from build123d import *

# Parameters (mm, degrees)
SKETCH1_W            = 32.9
SKETCH1_H            = 32.9
SKETCH1_W_2          = 20.2
SKETCH1_H_2          = 20.2
BOSS_EXTRUDE1_DEPTH  = 25
M4_CLEARANCE_HOLE1_D = 4.5
M4_CLEARANCE_HOLE2_D = 4.5
SKETCH8_W            = 32.9
SKETCH8_H            = 32.9
SKETCH8_W_2          = 20.2
SKETCH8_H_2          = 20.2
BOSS_EXTRUDE2_DEPTH  = 12.7
SKETCH9_W            = 87.4
SKETCH9_H            = 82.4
BOSS_EXTRUDE3_DEPTH  = 6.35
M2_CLEARANCE_HOLE1_D = 2.4
SKETCH13_W           = 20.2
SKETCH13_H           = 20.2
CUT_EXTRUDE1_DEPTH   = 71.911353111
SKETCH14_W           = 87.4
SKETCH14_H           = 82.4
CUT_EXTRUDE2_DEPTH   = 75.481759512
SKETCH15_W           = 35
SKETCH15_H           = 35
SKETCH15_R           = 1.625
BOSS_EXTRUDE4_DEPTH  = 6.35
FILLET1_R            = 6.35
SKETCH16_W           = 8
SKETCH16_H           = 22
CUT_EXTRUDE3_DEPTH   = 95.077926699
FILLET2_R            = 3.175


with BuildPart() as part:
    # Sketch1 → Boss-Extrude1 (new body)
    with BuildSketch(Plane(origin=(0, 0, 0), x_dir=(1, 0, 0), z_dir=(0, 1, 0))):
        Rectangle(SKETCH1_W, SKETCH1_H)
        Rectangle(SKETCH1_W_2, SKETCH1_H_2, mode=Mode.SUBTRACT)
    extrude(amount=BOSS_EXTRUDE1_DEPTH)

    # M4 Clearance Hole1 (through all)
    with Locations(Plane.XY.offset(16.45)):
        with Locations((0, 12.5)):
            Hole(M4_CLEARANCE_HOLE1_D / 2)

    # M4 Clearance Hole2 (through all)
    with Locations(Plane(origin=(16.45, 0, 0), x_dir=(0, 0, -1), z_dir=(1, 0, 0))):
        with Locations((0, 12.5)):
            Hole(M4_CLEARANCE_HOLE2_D / 2)

    # Sketch8 → Boss-Extrude2 (add)
    with BuildSketch(Plane(origin=(0, 25, 0), x_dir=(1, 0, 0), z_dir=(0, 1, 0))):
        Rectangle(SKETCH8_W, SKETCH8_H)
        Rectangle(SKETCH8_W_2, SKETCH8_H_2, mode=Mode.SUBTRACT)
    extrude(amount=BOSS_EXTRUDE2_DEPTH)

    # Sketch9 → Boss-Extrude3 (add)
    with BuildSketch(Plane(origin=(0, 37.7, 0), x_dir=(1, 0, 0), z_dir=(0, 1, 0))):
        Rectangle(SKETCH9_W, SKETCH9_H)
    extrude(amount=BOSS_EXTRUDE3_DEPTH)

    # M2 Clearance Hole1 (through all)
    with Locations(Plane(origin=(0, 44.05, 0), x_dir=(1, 0, 0), z_dir=(0, 1, 0))):
        with Locations((35, -25), (-22, -31), (-22, 31), (35, 25)):
            Hole(M2_CLEARANCE_HOLE1_D / 2)

    # Sketch13 → Cut-Extrude1 (cut, through all)
    with BuildSketch(Plane.XZ.offset(-37.7)):
        Rectangle(SKETCH13_W, SKETCH13_H)
    extrude(amount=-CUT_EXTRUDE1_DEPTH, mode=Mode.SUBTRACT)

    # Sketch14 → Cut-Extrude2 (cut, through all)
    with BuildSketch(Plane(origin=(0, 44.05, 0), x_dir=(1, 0, 0), z_dir=(0, 1, 0))):
        Rectangle(SKETCH14_W, SKETCH14_H)
        with BuildLine():
            Line((40, 23.784646643), (40, -23.784646643))
            ThreePointArc((40, -23.784646643), (38.369303562, -28.033255108), (34.314748382, -30.099756269))
            Line((34.314748382, -30.099756269), (-19.985251618, -35.815545743))
            ThreePointArc((-19.985251618, -35.815545743), (-24.898608465, -34.219739679), (-27, -29.500436117))
            Line((-27, -29.500436117), (-27, 29.500436117))
            ThreePointArc((-27, 29.500436117), (-24.898608465, 34.219739679), (-19.985251618, 35.815545743))
            Line((-19.985251618, 35.815545743), (34.314748382, 30.099756269))
            ThreePointArc((34.314748382, 30.099756269), (38.369303562, 28.033255108), (40, 23.784646643))
        make_face(mode=Mode.SUBTRACT)
    extrude(amount=-CUT_EXTRUDE2_DEPTH, mode=Mode.SUBTRACT)

    # Sketch15 → Boss-Extrude4 (add)
    with BuildSketch(Plane(origin=(0, 44.05, 0), x_dir=(1, 0, 0), z_dir=(0, 1, 0))):
        with Locations((57.5, 0)):
            Rectangle(SKETCH15_W, SKETCH15_H)
        with Locations(Location((65, 7.5, 0), (0, 0, 270))):
            Circle(SKETCH15_R, mode=Mode.SUBTRACT)
        with Locations(Location((65, -7.5, 0), (0, 0, 270))):
            Circle(SKETCH15_R, mode=Mode.SUBTRACT)
    extrude(amount=-BOSS_EXTRUDE4_DEPTH)

    # Fillet1
    fillet1_edges = [part.edges().sort_by_distance(p)[0] for p in [
        (40, 40.875, 17.5),
        (40, 40.875, -17.5),
    ]]
    fillet(fillet1_edges, radius=FILLET1_R)

    # Sketch16 → Cut-Extrude3 (cut, through all)
    with BuildSketch(Plane(origin=(0, 44.05, 0), x_dir=(1, 0, 0), z_dir=(0, 1, 0))):
        with Locations((49, 0)):
            Rectangle(SKETCH16_W, SKETCH16_H)
    extrude(amount=-CUT_EXTRUDE3_DEPTH, mode=Mode.SUBTRACT)

    # Fillet2
    fillet2_edges = [part.edges().sort_by_distance(p)[0] for p in [
        (45, 40.875, 11),
        (45, 40.875, -11),
        (53, 40.875, -11),
        (53, 40.875, 11),
    ]]
    fillet(fillet2_edges, radius=FILLET2_R)


solid = part.part
Model file for the job. Use its own axes, mm. A direction names the side the tool comes from. Give positions to 0.01 mm unless a question says otherwise; leave off trailing zeros. Loops run counter-clockwise (first coordinate to the right, second up) from the corner with the lowest first, then second, coordinate; pieces in that order, holes last. Notation, with made-up numbers: (83, 13) -> (117, 13) arc R29 cw to (117, 51) -> close; hole circle Ø6 at (-26.5, 69.25). An arc over 180 degrees is marked (long way). Use a Markdown table: item, result. Add a question column.
(1) Slice it at D-D on x = -6. List the corners of the cut face in (y, z), and give its area (3 significant figures).
(2) Slice it at B-B on x = 65. List the corners of the cut face in (y, z) (3 decimals).
(3) Tool access for faces 4 (the flat face through (0, 19, -16.45)), 5 (the cylindrical face through (-13.32, 14.73, -0.29)), 6 (the flat face through (0, 22, -10.1)): list every direction of +Z, -Z, +X, -X, +Y, -Y with a clear straight run to the whole face (end or side of a thin tool).
(4) Slice it at A-A on y = 27.5. List the corners of the cut face in (x, z).
(5) Mould opens along Z. For faces 1 (the cylindrical face through (34.446, 40.831, -23.935)), 2 (the flat face through (60, 41, -17.5)), 3 (the flat face through (60, 41, 17.5)) say: +Z half, -Z half, draft (parallel to the pull), parting line (faces both ways), or undercut.
(6) Drop flat-ended pins along their axis: pin 1 Ø8 at (x, z) = (58, -4) entering from -Y; pin 2 Ø10 at (x, y) = (-2, 17.5) entering from +Z; pin 3 Ø1.8 at (x, y) = (49, 41.5) entering from +Z; pin 4 Ø2.5 at (x, z) = (65, -7.5) entering from +Y. Give the stop position or say it passes through.
(7) Wall check: line 1 along Z through (x, y) = (35, 39); line 2 along X through (y, z) = (13.5, -4); line 3 along Y through (x, z) = (15.25, 0). Give the ranges that are in metal, low to high.
(8) Slice it at C-C on z = -25. List the corners of the cut face in (x, y).
Filled sheet:
| question | item | result |
|---|---|---|
| 1 | outline | (0, -16.45) -> (37.7, -16.45) -> (37.7, -34.34) -> (44.05, -34.34) -> (44.05, -10.1) -> (0, -10.1) -> close; (0, 10.1) -> (44.05, 10.1) -> (44.05, 34.34) -> (37.7, 34.34) -> (37.7, 16.45) -> (0, 16.45) -> close |
| 1 | area | 787 mm2 |
| 2 | outline | (37.7, -17.5) -> (44.05, -17.5) -> (44.05, -9.125) -> (37.7, -9.125) -> close; (37.7, -5.875) -> (44.05, -5.875) -> (44.05, 5.875) -> (37.7, 5.875) -> close; (37.7, 9.125) -> (44.05, 9.125) -> (44.05, 17.5) -> (37.7, 17.5) -> close |
| 3 | face 4 | -Z, +X, -X, -Y |
| 3 | face 5 | +X, -X |
| 3 | face 6 | +Y, -Y |
| 4 | outline | (-16.45, -16.45) -> (16.45, -16.45) -> (16.45, 16.45) -> (-16.45, 16.45) -> close; hole (-10.1, -10.1) -> (10.1, -10.1) -> (10.1, 10.1) -> (-10.1, 10.1) -> close |
| 5 | face 1 | undercut |
| 5 | face 2 | -Z half |
| 5 | face 3 | +Z half |
| 6 | pin 1 | y = 37.7 |
| 6 | pin 2 | z = 16.45 |
| 6 | pin 3 | z = 17.5 |
| 6 | pin 4 | through |
| 7 | line 1 | -29.99 to -26.2, -23.8 to 23.8, 26.2 to 29.99 |
| 7 | line 2 | -16.45 to -10.1, 10.1 to 16.45 |
| 7 | line 3 | 0 to 10.25, 14.75 to 44.05 |
| 8 | outline | (-27, 37.7) -> (33.8, 37.7) -> (33.8, 44.05) -> (-27, 44.05) -> close; (36.2, 37.7) -> (39.88, 37.7) -> (39.88, 44.05) -> (36.2, 44.05) -> close |
